from build123d import *

# Parameters (mm, degrees)
BOSS_EXTRUDE1_DEPTH      = 5.75
BOSS_EXTRUDE1_DEPTH_BACK = 5.75
SKETCH1_W                = 29.6
SKETCH1_H                = 8.3
SKETCH1_R                = 2.25
CUT_EXTRUDE1_DEPTH       = 2.75
CUT_EXTRUDE1_DEPTH_BACK  = 2.9
SKETCH1_4_W              = 29.6
SKETCH1_4_H              = 8.3
SKETCH1_4_R              = 2.25
BOSS_EXTRUDE2_DEPTH      = 5.75
BOSS_EXTRUDE2_DEPTH_BACK = 25
BOSS_EXTRUDE3_START      = -25
SKETCH1_6_R              = 9.6
BOSS_EXTRUDE3_DEPTH      = 6
BOSS_EXTRUDE5_START      = -25
SKETCH1_8_W              = 9
SKETCH1_8_H              = 30
BOSS_EXTRUDE5_DEPTH      = 36
BOSS_EXTRUDE6_START      = -25
SKETCH1_10_W             = 9
SKETCH1_10_H             = 30
BOSS_EXTRUDE6_DEPTH      = 32.5
CUT_EXTRUDE3_START       = -1
SKETCH5_R                = 11.1
SKETCH5_R_2              = 7
CUT_EXTRUDE3_DEPTH       = 8
SKETCH5_4_R              = 7
CUT_EXTRUDE4_DEPTH       = 108.001168218
CHAMFER1_SIZE            = 5
BOSS_EXTRUDE7_START      = -31
SKETCH1_17_R             = 12.6
SKETCH1_17_R_2           = 9.6
SKETCH1_17_R_3           = 7
BOSS_EXTRUDE7_DEPTH      = 17.3
CUT_EXTRUDE7_START       = -13.7
SKETCH1_18_R             = 9.6
SKETCH1_18_R_2           = 7
CUT_EXTRUDE7_DEPTH       = 5
BOSS_EXTRUDE8_START      = 6
BOSS_EXTRUDE8_DEPTH      = 5
BOSS_EXTRUDE9_START      = 11
SKETCH1_21_R             = 2.25
BOSS_EXTRUDE9_DEPTH      = 2
CUT_EXTRUDE5_START       = 46
SKETCH5_5_R              = 11.1
SKETCH5_5_R_2            = 2.2
CUT_EXTRUDE5_DEPTH       = 8
SKETCH6_R                = 12.8
CUT_EXTRUDE9_DEPTH       = 114.795869872
CUT_EXTRUDE10_START      = 20
SKETCH7_R                = 2.5
CUT_EXTRUDE10_DEPTH      = 94.795869872


with BuildPart() as part:
    # Sketch1 → Boss-Extrude1 (new, two sides: drawn at the far end of the back side and taken through both)
    with BuildSketch(Plane(origin=(0, 0, 0), x_dir=(1, 0, 0), z_dir=(0, 1, 0)).offset(-BOSS_EXTRUDE1_DEPTH_BACK)):
        with Locations((0, -0.45)):
            Rectangle(SKETCH1_W, SKETCH1_H)
        with Locations(Location((-10, 0, 0), (0, 0, 270))):
            Circle(SKETCH1_R, mode=Mode.SUBTRACT)
        with Locations(Location((10, 0, 0), (0, 0, 270))):
            Circle(SKETCH1_R, mode=Mode.SUBTRACT)
    extrude(amount=BOSS_EXTRUDE1_DEPTH + BOSS_EXTRUDE1_DEPTH_BACK)

    # Sketch1<4> → Cut-Extrude1 (cut, two sides: drawn at the far end of the back side and taken through both)
    with BuildSketch(Plane(origin=(0, 0, 0), x_dir=(1, 0, 0), z_dir=(0, 1, 0)).offset(-CUT_EXTRUDE1_DEPTH_BACK)):
        with Locations((0, -0.45)):
            Rectangle(SKETCH1_4_W, SKETCH1_4_H)
        with Locations(Location((-10, 0, 0), (0, 0, 270))):
            Circle(SKETCH1_4_R, mode=Mode.SUBTRACT)
        with Locations(Location((10, 0, 0), (0, 0, 270))):
            Circle(SKETCH1_4_R, mode=Mode.SUBTRACT)
    extrude(amount=CUT_EXTRUDE1_DEPTH + CUT_EXTRUDE1_DEPTH_BACK, mode=Mode.SUBTRACT)


with BuildPart() as cut_extrude1_piece_1:
    # of the separate pieces the step leaves, piece 1, a body of its own (cut_extrude1_pieces)
    add(part.part.solids().sort_by_distance((-14.8, 2.75, -3.7))[0])



with BuildPart() as cut_extrude1_piece_2:
    # of the separate pieces the step leaves, piece 2, a body of its own (cut_extrude1_pieces)
    add(part.part.solids().sort_by_distance((-14.8, -5.75, -3.7))[0])


with BuildPart() as cut_extrude1_piece_1_1:
    add(cut_extrude1_piece_1.part)

    add(cut_extrude1_piece_2.part)  # Boss-Extrude2 merges Cut-Extrude1 piece 2
    # Sketch1<5> → Boss-Extrude2 (add, two sides: drawn at the far end of the back side and taken through both)
    with BuildSketch(Plane(origin=(0, 0, 0), x_dir=(1, 0, 0), z_dir=(0, 1, 0)).offset(-BOSS_EXTRUDE2_DEPTH_BACK)):
        Polygon((14.8, -4.6), (-14.8, -4.6), (-20.8, -4.6), (-27, -8.6), (25.8, -8.6), (20.8, -4.6), align=None)
    extrude(amount=BOSS_EXTRUDE2_DEPTH + BOSS_EXTRUDE2_DEPTH_BACK)

    # Sketch1<6> → Boss-Extrude3 (add)
    with BuildSketch(Plane(origin=(0, 0, 0), x_dir=(1, 0, 0), z_dir=(0, 1, 0)).offset(BOSS_EXTRUDE3_START)):
        Polygon((-20.8, -4.6), (-27, -8.6), (-27, -91.5), (-17, -91.5), (-10, -80), (28, -80), (28, -50), (25.8, -8.6), (20.8, -4.6), align=None)
        with Locations(Location((0, -34, 0), (0, 0, 270))):
            Circle(SKETCH1_6_R, mode=Mode.SUBTRACT)
    extrude(amount=-BOSS_EXTRUDE3_DEPTH)

    # Sketch1<8> → Boss-Extrude5 (add)
    with BuildSketch(Plane(origin=(0, 0, 0), x_dir=(1, 0, 0), z_dir=(0, 1, 0)).offset(BOSS_EXTRUDE5_START)):
        Polygon((-24, -42.5), (-27, -42.5), (-27, -91.5), (-17, -91.5), (-14.565217391, -87.5), (-24, -87.5), align=None)
        with Locations((23.5, -65)):
            Rectangle(SKETCH1_8_W, SKETCH1_8_H)
    extrude(amount=BOSS_EXTRUDE5_DEPTH)

    # Sketch1<10> → Boss-Extrude6 (add)
    with BuildSketch(Plane(origin=(0, 0, 0), x_dir=(1, 0, 0), z_dir=(0, 1, 0)).offset(BOSS_EXTRUDE6_START)):
        with Locations((23.5, -65)):
            Rectangle(SKETCH1_10_W, SKETCH1_10_H)
    extrude(amount=BOSS_EXTRUDE6_DEPTH)

    # Sketch5 → Cut-Extrude3 (cut)
    # profile 1 of 2: a face of its own
    with BuildSketch(Plane.ZY.offset(-19).offset(CUT_EXTRUDE3_START)):
        with Locations((65, -8.5)):
            Circle(SKETCH5_R)
        with Locations((65, -8.5)):
            Circle(SKETCH5_R_2, mode=Mode.SUBTRACT)
    # profile 2 of 2: a face of its own
    with BuildSketch(Plane.ZY.offset(-19).offset(CUT_EXTRUDE3_START)):
        with Locations((65, -8.5)):
            Circle(SKETCH5_R_2)
    extrude(amount=-CUT_EXTRUDE3_DEPTH, mode=Mode.SUBTRACT)

    # Sketch5<4> → Cut-Extrude4 (cut, through all)
    with BuildSketch(Plane.ZY.offset(-19)):
        with Locations((65, -8.5)):
            Circle(SKETCH5_4_R)
    extrude(amount=-CUT_EXTRUDE4_DEPTH, mode=Mode.SUBTRACT)

    # Chamfer1
    chamfer1_edges = [cut_extrude1_piece_1_1.edges().sort_by_distance(p)[0] for p in [
        (-0.6, -25, 8.6),
    ]]
    chamfer(chamfer1_edges, length=CHAMFER1_SIZE)

    # Sketch1<17> → Boss-Extrude7 (add)
    # profile 1 of 2: a face of its own
    with BuildSketch(Plane(origin=(0, 0, 0), x_dir=(1, 0, 0), z_dir=(0, 1, 0)).offset(BOSS_EXTRUDE7_START)):
        with Locations(Location((0, -34, 0), (0, 0, 270))):
            Circle(SKETCH1_17_R)
        with Locations((0, -34)):
            Circle(SKETCH1_17_R_2, mode=Mode.SUBTRACT)
    # profile 2 of 2: a face of its own
    with BuildSketch(Plane(origin=(0, 0, 0), x_dir=(1, 0, 0), z_dir=(0, 1, 0)).offset(BOSS_EXTRUDE7_START)):
        with Locations((0, -34)):
            Circle(SKETCH1_17_R_2)
        with Locations(Location((0, -34, 0), (0, 0, 270))):
            Circle(SKETCH1_17_R_3, mode=Mode.SUBTRACT)
    extrude(amount=BOSS_EXTRUDE7_DEPTH)

    # Sketch1<18> → Cut-Extrude7 (cut)
    with BuildSketch(Plane(origin=(0, 0, 0), x_dir=(1, 0, 0), z_dir=(0, 1, 0)).offset(CUT_EXTRUDE7_START)):
        with Locations(Location((0, -34, 0), (0, 0, 270))):
            Circle(SKETCH1_18_R)
        with Locations(Location((0, -34, 0), (0, 0, 270))):
            Circle(SKETCH1_18_R_2, mode=Mode.SUBTRACT)
    extrude(amount=-CUT_EXTRUDE7_DEPTH, mode=Mode.SUBTRACT)

    # Sketch1<20> → Boss-Extrude8 (add)
    # profile 1 of 2: a face of its own
    with BuildSketch(Plane(origin=(0, 0, 0), x_dir=(1, 0, 0), z_dir=(0, 1, 0)).offset(BOSS_EXTRUDE8_START)):
        with BuildLine():
            Line((35, -50), (28, -50))
            Line((28, -50), (28, -80))
            Line((28, -80), (35, -80))
            ThreePointArc((35, -80), (37.474873734, -78.974873734), (38.5, -76.5))
            Line((38.5, -76.5), (38.5, -53.5))
            ThreePointArc((38.5, -53.5), (37.474873734, -51.025126266), (35, -50))
        make_face()
        Polygon((32.75, -78.330127019), (29, -76.165063509), (29, -71.834936491), (32.75, -69.669872981), (36.5, -71.834936491), (36.5, -76.165063509), align=None, mode=Mode.SUBTRACT)
        Polygon((36.5, -58.165063509), (32.75, -60.330127019), (29, -58.165063509), (29, -53.834936491), (32.75, -51.669872981), (36.5, -53.834936491), align=None, mode=Mode.SUBTRACT)
    # profile 2 of 2: a face of its own
    with BuildSketch(Plane(origin=(0, 0, 0), x_dir=(1, 0, 0), z_dir=(0, 1, 0)).offset(BOSS_EXTRUDE8_START)):
        with BuildLine():
            Line((-17, -91.5), (-27, -91.5))
            Line((-27, -91.5), (-27, -97.5))
            ThreePointArc((-27, -97.5), (-22, -102.5), (-17, -97.5))
            Line((-17, -97.5), (-17, -91.5))
        make_face()
        Polygon((-19.834936491, -92.5), (-17.669872981, -96.25), (-19.834936491, -100), (-24.165063509, -100), (-26.330127019, -96.25), (-24.165063509, -92.5), align=None, mode=Mode.SUBTRACT)
    extrude(amount=BOSS_EXTRUDE8_DEPTH)

    # Sketch1<21> → Boss-Extrude9 (add)
    # profile 1 of 3: a face of its own
    with BuildSketch(Plane(origin=(0, 0, 0), x_dir=(1, 0, 0), z_dir=(0, 1, 0)).offset(BOSS_EXTRUDE9_START)):
        Polygon((29, -53.834936491), (29, -58.165063509), (32.75, -60.330127019), (36.5, -58.165063509), (36.5, -53.834936491), (32.75, -51.669872981), align=None)
        with Locations(Location((32.75, -56, 0), (0, 0, 270))):
            Circle(SKETCH1_21_R, mode=Mode.SUBTRACT)
    # profile 2 of 3: a face of its own
    with BuildSketch(Plane(origin=(0, 0, 0), x_dir=(1, 0, 0), z_dir=(0, 1, 0)).offset(BOSS_EXTRUDE9_START)):
        Polygon((32.75, -69.669872981), (29, -71.834936491), (29, -76.165063509), (32.75, -78.330127019), (36.5, -76.165063509), (36.5, -71.834936491), align=None)
        with Locations(Location((32.75, -74, 0), (0, 0, 270))):
            Circle(SKETCH1_21_R, mode=Mode.SUBTRACT)
    # profile 3 of 3: a face of its own
    with BuildSketch(Plane(origin=(0, 0, 0), x_dir=(1, 0, 0), z_dir=(0, 1, 0)).offset(BOSS_EXTRUDE9_START)):
        Polygon((-24.165063509, -100), (-19.834936491, -100), (-17.669872981, -96.25), (-19.834936491, -92.5), (-24.165063509, -92.5), (-26.330127019, -96.25), align=None)
        with Locations(Location((-22, -96.25, 0), (0, 0, 270))):
            Circle(SKETCH1_21_R, mode=Mode.SUBTRACT)
    extrude(amount=-BOSS_EXTRUDE9_DEPTH)

    # Sketch5<5> → Cut-Extrude5 (cut)
    with BuildSketch(Plane.ZY.offset(-19).offset(CUT_EXTRUDE5_START)):
        with Locations((65, -8.5)):
            Circle(SKETCH5_5_R)
        with Locations((52.272077939, 4.227922061)):
            Circle(SKETCH5_5_R_2)
        with Locations((77.727922061, 4.227922061)):
            Circle(SKETCH5_5_R_2)
        with Locations((77.727922061, -21.227922061)):
            Circle(SKETCH5_5_R_2)
        with Locations((52.272077939, -21.227922061)):
            Circle(SKETCH5_5_R_2)
    extrude(amount=-CUT_EXTRUDE5_DEPTH, mode=Mode.SUBTRACT)

    # Sketch6 → Cut-Extrude9 (cut, through all)
    with BuildSketch(Plane(origin=(0, 0, 0), x_dir=(0, 0, -1), z_dir=(1, 0, 0))):
        with Locations((-65, -8.5)):
            Circle(SKETCH6_R)
    extrude(amount=-CUT_EXTRUDE9_DEPTH, mode=Mode.SUBTRACT)

    # Sketch7 → Cut-Extrude10 (cut, through all)
    with BuildSketch(Plane.XY.offset(CUT_EXTRUDE10_START)):
        with Locations(Location((-21, -8.5, 0), (0, 0, 180))):
            Circle(SKETCH7_R)
    extrude(amount=CUT_EXTRUDE10_DEPTH, mode=Mode.SUBTRACT)


solid = cut_extrude1_piece_1_1.part
Read the model definition and answer for the solid it produces. Units are mm, in the model's axes. A direction names the side the tool comes from. Give positions to 0.01 mm unless a question says otherwise; leave off trailing zeros. Loops run counter-clockwise (first coordinate to the right, second up) from the corner with the lowest first, then second, coordinate; pieces in that order, holes last. Notation, with made-up numbers: (7, -6.75) -> (42, -6.75) arc R6 ccw to (42, 4.25) -> close; hole circle Ø6 at (44.5, -38.5). An arc over 180 degrees is marked (long way). Use a Markdown table: item, result.
Q1. Each of these flat-tipped pins is pushed along its axis until it touches: pin 1 (3.5 mm diameter, centred on x = -10, z = 0, fed in from +Y); pin 2 (3.5 mm diameter, centred on x = -21.5, y = 8, fed in from -Z); pin 3 (1.5 mm diameter, centred on x = -19, z = 68, fed in from +Y); pin 4 (18 mm diameter, centred on x = 0, z = 34, fed in from +Y). Where does it stop, or does it pass through?
Solved:
| item | result |
|---|---|
| pin 1 | passes through |
| pin 2 | stops at z = 87.5 |
| pin 3 | stops at y = -25 |
| pin 4 | stops at y = -18.7 |
Q2. Find the intervals of material crossed by line 1 along X through (y, z) = (10, 74); line 2 along X through (y, z) = (10.1, 96.25); line 3 along Y through (x, z) = (25.5, 21), in increasing order.
Solved:
| item | result |
|---|---|
| line 1 | x = -27 to -24, 19 to 30.5, 35 to 38.5 |
| line 2 | x = -27 to -24.25, -19.75 to -17 |
| line 3 | y = -31 to -25 |
Q3. Section D-D, the plane y = -17 is taken. Determine the outline of the cut face in (x, z).
Solved:
| item | result |
|---|---|
| outline | (-27, 8.6) -> (-20.8, 4.6) -> (20.8, 4.6) -> (25.8, 8.6) -> close; (-27, 42.5) -> (-24, 42.5) -> (-24, 55.43) -> (-27, 55.43) -> close; (-27, 74.57) -> (-24, 74.57) -> (-24, 87.5) -> (-14.57, 87.5) -> (-17, 91.5) -> (-27, 91.5) -> close; circle Ø25.2 at (0, 34); (19, 50) -> (28, 50) -> (28, 57.86) -> (20, 57.86) -> (20, 72.14) -> (28, 72.14) -> (28, 80) -> (19, 80) -> close; hole circle Ø19.2 at (0, 34) |
Q4. Section C-C, the plane z = 65 is taken. Determine the outline of the cut face in (x, y), then the cut area to 3 significant figures.
Solved:
| item | result |
|---|---|
| outline | (-27, -31) -> (28, -31) -> (28, -19.6) -> (20, -19.6) -> (20, -15.5) -> (19, -15.5) -> (19, -25) -> (-24, -25) -> (-24, -21.3) -> (-27, -21.3) -> close; (-27, 4.3) -> (-24, 4.3) -> (-24, 11) -> (-27, 11) -> close; (19, -1.5) -> (20, -1.5) -> (20, 2.6) -> (28, 2.6) -> (28, 6) -> (38.5, 6) -> (38.5, 11) -> (19, 11) -> close |
| area | 546 mm^2 |
Q5. Section B-B, the plane z = 0 is taken. Determine the outline of the cut face in (x, y).
Solved:
| item | result |
|---|---|
| outline | (-14.8, -5.75) -> (-12.25, -5.75) -> (-12.25, -2.9) -> (-14.8, -2.9) -> close; (-14.8, 2.75) -> (-12.25, 2.75) -> (-12.25, 5.75) -> (-14.8, 5.75) -> close; (-7.75, -5.75) -> (7.75, -5.75) -> (7.75, -2.9) -> (-7.75, -2.9) -> close; (-7.75, 2.75) -> (7.75, 2.75) -> (7.75, 5.75) -> (-7.75, 5.75) -> close; (12.25, -5.75) -> (14.8, -5.75) -> (14.8, -2.9) -> (12.25, -2.9) -> close; (12.25, 2.75) -> (14.8, 2.75) -> (14.8, 5.75) -> (12.25, 5.75) -> close |
Q6. A tool of negligible diameter and unlimited length cuts with its end or side. For faces 1 (the face through (23.94, -8.01, 53.91)), 2 (the face through (-25.52, -20.57, 54.37)), 3 (the face through (30.9, 7.48, 59.26)), from which of +Z, -Z, +X, -X, +Y, -Y can it reach the whole face along a straight path? Write none if from no direction.
Solved:
| item | result |
|---|---|
| face 1 | +X |
| face 2 | -X |
| face 3 | -Y |
Q7. Determine the mould class of faces 4 (the face through (-22, -13, 91.5)), 5 (the face through (29, 7, 74)), 6 (the face through (38.5, 8, 65)) for opening direction Z: pulls with the +Z half, pulls with the -Z half, needs draft (parallel to the pull), parting line crosses it, or undercut.
Solved:
| item | result |
|---|---|
| face 4 | pulls with the +Z half |
| face 5 | undercut |
| face 6 | needs draft |
Q8. Section A-A, the plane y = -8.5 is taken. Count the separate pieces of the cut face and the enclosed holes in it, then the cut area to 3 significant figures.
Solved:
| item | result |
|---|---|
| separate pieces | 6 |
| enclosed holes | 0 |
| area | 350 mm^2 |
